```python
from build123d import *

# Parameters (mm, degrees)
F0_W     = 49.53
F0_H     = 45.72
F1_DEPTH = 35.0012
F3_R     = 3.1877
F4_DEPTH = 35.0022
F3_R_2   = 3.3655
F5_DEPTH = 35.0022
F6_SIZE  = 0.508


with BuildPart() as f1:
    # F0 (on Front) → F1 (new body)
    with BuildSketch(Plane.XZ):
        with Locations((0, -3.515769)):
            Rectangle(F0_W, F0_H)
    extrude(amount=F1_DEPTH)

    # F3 (on face) → F4 (cut, through all)
    with BuildSketch(Plane.XZ.offset(35.0012)):
        with Locations((-15.875, 11.775031)):
            Circle(F3_R)
        with Locations((15.875, 11.775031)):
            Circle(F3_R)
    extrude(amount=-F4_DEPTH, mode=Mode.SUBTRACT)

    # F3 (on face) → F5 (cut, through all)
    with BuildSketch(Plane.XZ.offset(35.0012)):
        with Locations((0, 11.775031)):
            Circle(F3_R_2)
    extrude(amount=-F5_DEPTH, mode=Mode.SUBTRACT)

    # F6
    f6_edges = [f1.edges().sort_by_distance(p)[0] for p in [
        (-3.3655, 0, 11.775031),
        (12.6873, -35.0012, 11.775031),
        (-3.3655, -35.0012, 11.775031),
        (-19.0627, -35.0012, 11.775031),
        (12.6873, 0, 11.775031),
        (-19.0627, 0, 11.775031),
    ]]
    chamfer(f6_edges, length=F6_SIZE)


solid = f1.part
```
Input: part model. Units: mm. Frame: model coordinates. Coordinates: 2 decimals unless noted, no trailing zeros. Write each loop counter-clockwise with the first axis right and the second up, starting at its lowest first coordinate (ties: lowest second). Pieces come first, ordered by that corner, then holes.
1) Pin query (flat end, axial travel): pin 1 Ø5 at (x, z) = (15.88, 11.78) entering from +Y. Return the tip coordinate at first contact, or that it passes through.
2) Mould query, pull axis Z, two halves, no side actions, for faces 1 (the cylindrical face through (18.915, -17.738, 12.733)), 2 (the flat face through (24.765, -17, -4)), 3 (the flat face through (0, -17, 19.344)), 4 (the flat face through (0, -17, -26.376)). Classes: pulls with the +Z half, pulls with the -Z half, needs draft (parallel to the pull), parting line crosses it, or undercut.
3) Section B-B on y = -8. Output: boundary loops of the cut face in (x, z) (1 decimal), and give its area (3 significant figures).
4) Section A-A on x = 0. Output: boundary loops of the cut face in (y, z).
5) Material intervals for line 1 along X through (y, z) = (-26, 11.5) (3 decimals); line 2 along X through (y, z) = (-12.5, 14) (3 decimals); line 3 along Z through (x, y) = (15, -28.5), sorted ascending.
Check result:
1. pin 1: passes through
2. face 1: undercut
2. face 2: needs draft
2. face 3: pulls with the +Z half
2. face 4: pulls with the -Z half
3. outline: (-24.8, -26.4) - (24.8, -26.4) - (24.8, 19.3) - (-24.8, 19.3) - close; hole circle Ø6.4 at (-15.9, 11.8); hole circle Ø6.7 at (0, 11.8); hole circle Ø6.4 at (15.9, 11.8)
3. area: 2,170 mm2
4. outline: (-35, -26.38) - (0, -26.38) - (0, 7.9) - (-0.51, 8.41) - (-34.49, 8.41) - (-35, 7.9) - close; (-35, 15.65) - (-34.49, 15.14) - (-0.51, 15.14) - (0, 15.65) - (0, 19.34) - (-35, 19.34) - close
5. line 1: x = -24.765 to -19.051, -12.699 to -3.354, 3.354 to 12.699, 19.051 to 24.765
5. line 2: x = -24.765 to -18.158, -13.592 to -2.525, 2.525 to 13.592, 18.158 to 24.765
5. line 3: z = -26.38 to 8.71, 14.84 to 19.34
